Read the model definition and answer for the solid it produces. Units are mm, in the model's axes. Round coordinates to 2 decimals unless told otherwise and drop trailing zeros. Write each loop counter-clockwise with the first axis right and the second up, starting at its lowest first coordinate (ties: lowest second). Pieces come first, ordered by that corner, then holes. Notation, with made-up numbers: (-36, 11.25) - (-10, 11.25) arc R16 ccw to (-10, 18.25) - close; hole circle Ø11 at (0.5, 30). An arc over 180 degrees is marked (long way). One line per item, written item: value. Start each with the question number.
(1) The mould has two halves that part along Y. Classify faces 1 (the face through (86.478, 59.966, 0.74)), 2 (the face through (49, 33, 1.5)): +Y half, -Y half, draft (parallel to the pull), parting line (faces both ways), or undercut.
(2) Find the intervals of material crossed by L1, parallel to Y at x = 97.5, z = 1; L2, parallel to Y at x = 88, z = 0.5; L3, parallel to Y at x = 85, z = 0.3, in increasing order.
(3) A cutting plane is placed at B-B, the plane x = 17.5. Determine the outline of the cut face in (y, z).
(4) A cutting plane is placed at C-C, the plane y = 51.5. Determine the outline of the cut face in (x, z).
(5) Flat-ended cylindrical pins translate along their axes: pin 1 Ø3 at (x, y) = (17.5, 51.5) entering from -Z; pin 2 Ø4 at (x, y) = (17.5, 2.5) entering from +Z. Find the tip coordinate at first contact, or state that the pin passes through.
(6) A cutting plane is placed at A-A, the plane y = 59.5. Determine the outline of the cut face in (x, z), plus the area to 3 significant figures.
(7) A cutting plane is placed at D-D, the plane x = 75. Determine the outline of the cut face in (y, z).
from build123d import *

# Parameters (mm, degrees)
SKETCH_1_W      = 100
SKETCH_1_H      = 65
SKETCH_1_R      = 1.55
EXTRUDE_1_DEPTH = 1.5


with BuildPart() as part:
    # Эскиз1 → Бобышка-Вытянуть1 (new body)
    with BuildSketch(Plane.XY):
        with Locations((50, 32.5)):
            Rectangle(SKETCH_1_W, SKETCH_1_H)
        with Locations((17.5, 51.5)):
            Circle(SKETCH_1_R, mode=Mode.SUBTRACT)
        with Locations((97.5, 51.5)):
            Circle(SKETCH_1_R, mode=Mode.SUBTRACT)
        with Locations((97.5, 2.5)):
            Circle(SKETCH_1_R, mode=Mode.SUBTRACT)
        with Locations((17.5, 2.5)):
            Circle(SKETCH_1_R, mode=Mode.SUBTRACT)
        with Locations((85, 59.5)):
            Circle(SKETCH_1_R, mode=Mode.SUBTRACT)
        with BuildLine():
            Line((63, 30), (93, 30))
            ThreePointArc((93, 30), (93.707106781, 29.707106781), (94, 29))
            Line((94, 29), (94, 22))
            ThreePointArc((94, 22), (93.707106781, 21.292893219), (93, 21))
            Line((93, 21), (63, 21))
            ThreePointArc((63, 21), (62.292893219, 21.292893219), (62, 22))
            Line((62, 22), (62, 29))
            ThreePointArc((62, 29), (62.292893219, 29.707106781), (63, 30))
        make_face(mode=Mode.SUBTRACT)
    extrude(amount=EXTRUDE_1_DEPTH)


solid = part.part
Here are the results:
1. face 1: undercut
1. face 2: draft
2. L1: 0 to 0.95, 4.05 to 49.95, 53.05 to 65
2. L2: 0 to 21, 30 to 65
2. L3: 0 to 21, 30 to 57.95, 61.05 to 65
3. outline: (0, 0) - (0.95, 0) - (0.95, 1.5) - (0, 1.5) - close; (4.05, 0) - (49.95, 0) - (49.95, 1.5) - (4.05, 1.5) - close; (53.05, 0) - (65, 0) - (65, 1.5) - (53.05, 1.5) - close
4. outline: (0, 0) - (15.95, 0) - (15.95, 1.5) - (0, 1.5) - close; (19.05, 0) - (95.95, 0) - (95.95, 1.5) - (19.05, 1.5) - close; (99.05, 0) - (100, 0) - (100, 1.5) - (99.05, 1.5) - close
5. pin 1: through
5. pin 2: z = 1.5
6. outline: (0, 0) - (83.45, 0) - (83.45, 1.5) - (0, 1.5) - close; (86.55, 0) - (100, 0) - (100, 1.5) - (86.55, 1.5) - close
6. area: 145 mm²
7. outline: (0, 0) - (21, 0) - (21, 1.5) - (0, 1.5) - close; (30, 0) - (65, 0) - (65, 1.5) - (30, 1.5) - close
